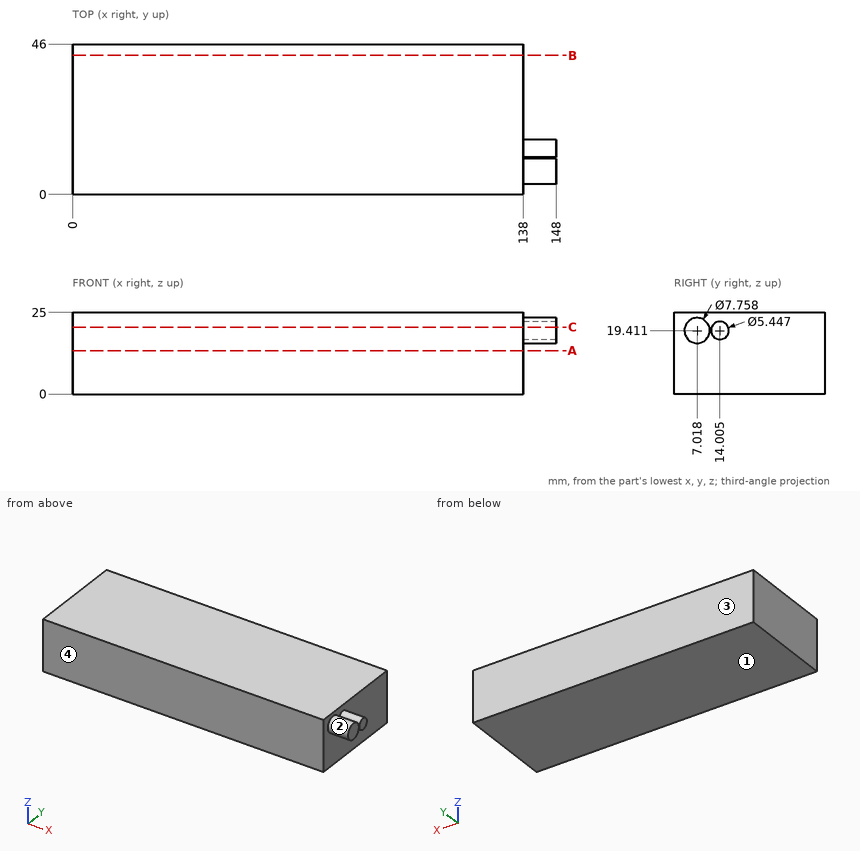
Part print with two shaded views. Sizes in mm from the minimum x, y, z corner. Round coordinates to 2 decimals unless told otherwise and drop trailing zeros. Order: outer loops, then holes, each group sorted by start corner. A loop starts at its lowest first (then second) coordinate and runs counter-clockwise, first axis right, second up.
(1) Drill centre lines: line 1 (Y direction, x = 142.5, z = 19) (1 decimal); line 2 (X direction, y = 22.5, z = 8.25). Where is each one in solid material? Low to high.
(2) Band-saw the part on B-B (y = 42.5). List the corners of the cut face in (x, z).
(3) Band-saw the part on C-C (z = 20.5). List the corners of the cut face in (x, y) (1 decimal), then the cut area to 3 significant figures.
(4) Pull direction Y, two halves, no side cores. Call the marked faces 1, 2, 3 and 4: released by +Y, released by -Y, zero draft, split by the parting line, or undercut.
(5) Band-saw the part on A-A (z = 13.25). List the corners of the cut face in (x, y), then the cut area to 3 significant figures.
(6) Pin check, flat tip, straight feed: pin 1 (12 mm diameter, centred on y = 29.5, z = 20, fed in from +X). Stop position of the tip, or through.
Verdict:
1. line 1: y = 3.2 to 10.9, 11.3 to 16.7
1. line 2: x = 0 to 138
2. outline: (0, 0) - (138, 0) - (138, 25) - (0, 25) - close
3. outline: (0, 0) - (138, 0) - (138, 3.3) - (148, 3.3) - (148, 10.7) - (138, 10.7) - (138, 11.5) - (148, 11.5) - (148, 16.5) - (138, 16.5) - (138, 46) - (0, 46) - close
3. area: 6,470 mm2
4. face 1: zero draft
4. face 2: undercut
4. face 3: released by +Y
4. face 4: released by -Y
5. outline: (0, 0) - (138, 0) - (138, 46) - (0, 46) - close
5. area: 6,350 mm2
6. pin 1: stops at x = 138
